Check sheet for the modelled part. Datum: model origin and axes. Units: mm. Face numbers are marked on the shaded views. Give positions to 0.01 mm unless a question says otherwise; leave off trailing zeros. Write each loop counter-clockwise with the first axis right and the second up, starting at its lowest first coordinate (ties: lowest second). Pieces come first, ordered by that corner, then holes. Notation, with made-up numbers: M -27,-37 L 17,-37 A24 ccw 17,-15 Z; hole C 13,18 d7. An arc over 180 degrees is marked long. Write item = value, one per line. Start each with the question number.
1) Cross-section at B-B, the plane x = 0. Record the cut outline in (y, z).
2) Scan lines: line 1 along Z through (x, y) = (0, -65); line 2 along Y through (x, z) = (-100, 22); line 3 along X through (y, z) = (-236.5, 9.5). Record each from-to range of solid material in increasing order. Write a range as [from, to].
3) Cross-section at D-D, the plane z = 158.5. Record the cut outline in (x, y).
4) Go/stop test with flat-tipped pins: pin 1 (2 mm diameter, centred on x = 42.5, y = -137, fed in from +Z); pin 2 (10 mm diameter, centred on x = 76, y = -205.5, fed in from +Z); pin 3 (8 mm diameter, centred on x = 103.5, y = -68, fed in from -Z). Record where each tip stops, or that it passes through.
5) Mould release check, pull along X, two halves, no side actions. Record for the marked faces 1, 2 and 3: released by +X, released by -X, zero draft, split by the parting line, or undercut.
6) Cross-section at A-A, the plane z = 0. Record the cut outline in (x, y), plus the area to 3 significant figures.
7) Cross-section at C-C, the plane y = -42. Record the cut outline in (x, z), plus the area to 3 significant figures.
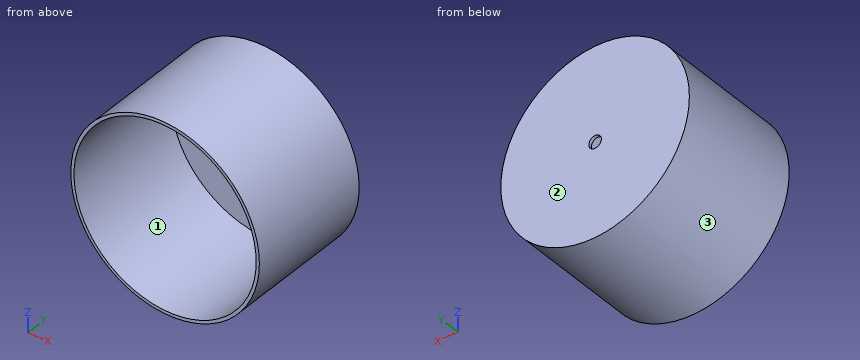
```python
from build123d import *

# Parameters (mm, degrees)
F0_R     = 190.5
F1_DEPTH = 254
F2_R     = 184.149995
F3_DEPTH = 247.65
F4_R     = 12.7
F5_DEPTH = 254.001


with BuildPart() as f1:
    # F0 (on Front) → F1 (new body)
    with BuildSketch(Plane.XZ):
        Circle(F0_R)
    extrude(amount=F1_DEPTH)

    # F2 (on face) → F3 (cut)
    with BuildSketch(Plane.XZ.offset(254)):
        Circle(F2_R)
    extrude(amount=-F3_DEPTH, mode=Mode.SUBTRACT)

    # F4 (on face) → F5 (cut, through all)
    with BuildSketch(Plane(origin=(0, 0, 0), x_dir=(-1, 0, 0), z_dir=(0, 1, 0))):
        Circle(F4_R)
    extrude(amount=-F5_DEPTH, mode=Mode.SUBTRACT)


solid = f1.part
```
Reply:
q1.outline = M -254,-190.5 L 0,-190.5 L 0,-12.7 L -6.35,-12.7 L -6.35,-184.15 L -254,-184.15 Z; M -254,184.15 L -6.35,184.15 L -6.35,12.7 L 0,12.7 L 0,190.5 L -254,190.5 Z
q2.line_1 = [-190.5, -184.15], [184.15, 190.5]
q2.line_2 = [-6.35, 0]
q2.line_3 = [-190.26, -183.9], [183.9, 190.26]
q3.outline = M -105.68,-254 L -93.75,-254 L -93.75,-6.35 L 93.75,-6.35 L 93.75,-254 L 105.68,-254 L 105.68,0 L -105.68,0 Z
q4.pin_1 = 185.92
q4.pin_2 = 176.77
q4.pin_3 = -162.45
q5.face_1 = undercut
q5.face_2 = zero draft
q5.face_3 = split by the parting line
q6.outline = M -190.5,-254 L -184.15,-254 L -184.15,-6.35 L -12.7,-6.35 L -12.7,0 L -190.5,0 Z; M 12.7,-6.35 L 184.15,-6.35 L 184.15,-254 L 190.5,-254 L 190.5,0 L 12.7,0 Z
q6.area = 5,400 mm2
q7.outline = C 0,0 d381; hole C 0,0 d368.3
q7.area = 7,470 mm2
